Source: CAD feature listing. Evaluate the final solid. Frame: model axes, mm. A direction names the side the tool comes from. Round coordinates to 2 decimals unless told otherwise and drop trailing zeros. Order: outer loops, then holes, each group sorted by start corner. A loop starts at its lowest first (then second) coordinate and runs counter-clockwise, first axis right, second up. Notation, with made-up numbers: (-1.75, -20.75) -> (6.25, -20.75) arc R29 cw to (6.25, -0.75) -> close; hole circle Ø11 at (-14.75, 73.5). An arc over 180 degrees is marked (long way). Answer as CSV lines item,"result".
from build123d import *

# Parameters (mm, degrees)
CYLINDER007_R               = 5
CYLINDER007_DEPTH           = 5
COMPOUND003_PLACEMENT_ANGLE = 119
CYLINDER008_R               = 5
CYLINDER008_DEPTH           = 6
COMPOUND004_PLACEMENT_ANGLE = 119
CYLINDER006_R               = 5
CYLINDER006_DEPTH           = 6
CYLINDER004_R               = 2.5
CYLINDER004_DEPTH           = 12
COMPOUND_PLACEMENT_ANGLE    = 119
CYLINDER005_R               = 2.5
CYLINDER005_DEPTH           = 12
COMPOUND001_PLACEMENT_ANGLE = 241
CYLINDER003_R               = 2.5
CYLINDER003_DEPTH           = 12
BOX_W                       = 200
BOX_H                       = 100
BOX_DEPTH                   = 12
CYLINDER001_R               = 37.5
CYLINDER001_DEPTH           = 3
CYLINDER002_R               = 41
CYLINDER002_DEPTH           = 3
CYLINDER_R                  = 50
CYLINDER_DEPTH              = 12


with BuildPart() as compound003:
    # Cylinder007 → Cylinder007 (new body)
    with BuildSketch(Plane(origin=(0, -43.5, 0), x_dir=(1, 0, 0), z_dir=(0, 0, 1))):
        Circle(CYLINDER007_R)
    extrude(amount=CYLINDER007_DEPTH)


with BuildPart() as compound003_1:
    # Compound003 placement: moved
    add(compound003.part.rotate(Axis((0, 0, 0), (0, 0, 1)), COMPOUND003_PLACEMENT_ANGLE))


with BuildPart() as compound004:
    # Cylinder008 → Cylinder008 (new body)
    with BuildSketch(Plane(origin=(0, -43.5, 0), x_dir=(1, 0, 0), z_dir=(0, 0, 1))):
        Circle(CYLINDER008_R)
    extrude(amount=CYLINDER008_DEPTH)


with BuildPart() as compound004_1:
    # Compound004 placement: moved
    add(compound004.part.rotate(Axis((0, 0, 0), (0, 0, -1)), COMPOUND004_PLACEMENT_ANGLE))


with BuildPart() as compound005:
    # Cylinder006 → Cylinder006 (new body)
    with BuildSketch(Plane(origin=(0, -43.5, 0), x_dir=(1, 0, 0), z_dir=(0, 0, 1))):
        Circle(CYLINDER006_R)
    extrude(amount=CYLINDER006_DEPTH)

    # Compound005: union Compound003, Compound004
    add(compound003_1.part)
    add(compound004_1.part)


with BuildPart() as compound:
    # Cylinder004 → Cylinder004 (new body)
    with BuildSketch(Plane(origin=(0, -43.5, 0), x_dir=(1, 0, 0), z_dir=(0, 0, 1))):
        Circle(CYLINDER004_R)
    extrude(amount=CYLINDER004_DEPTH)


with BuildPart() as compound_1:
    # Compound placement: moved
    add(compound.part.rotate(Axis((0, 0, 0), (0, 0, 1)), COMPOUND_PLACEMENT_ANGLE))


with BuildPart() as compound001:
    # Cylinder005 → Cylinder005 (new body)
    with BuildSketch(Plane(origin=(0, -43.5, 0), x_dir=(1, 0, 0), z_dir=(0, 0, 1))):
        Circle(CYLINDER005_R)
    extrude(amount=CYLINDER005_DEPTH)


with BuildPart() as compound001_1:
    # Compound001 placement: moved
    add(compound001.part.rotate(Axis((0, 0, 0), (0, 0, 1)), COMPOUND001_PLACEMENT_ANGLE))


with BuildPart() as compound002:
    # Cylinder003 → Cylinder003 (new body)
    with BuildSketch(Plane(origin=(0, -43.5, 0), x_dir=(1, 0, 0), z_dir=(0, 0, 1))):
        Circle(CYLINDER003_R)
    extrude(amount=CYLINDER003_DEPTH)

    # Compound002: union Compound, Compound001
    add(compound_1.part)
    add(compound001_1.part)


with BuildPart() as cube:
    # Box → Box (new body)
    with BuildSketch(Plane(origin=(-100, 44, 0), x_dir=(1, 0, 0), z_dir=(0, 0, 1))):
        with Locations((100, 50)):
            Rectangle(BOX_W, BOX_H)
    extrude(amount=BOX_DEPTH)


with BuildPart() as cylinder001:
    # Cylinder001 → Cylinder001 (new body)
    with BuildSketch(Plane.XY):
        Circle(CYLINDER001_R)
    extrude(amount=CYLINDER001_DEPTH)


with BuildPart() as cut:
    # Cylinder002 → Cylinder002 (new body)
    with BuildSketch(Plane.XY):
        Circle(CYLINDER002_R)
    extrude(amount=CYLINDER002_DEPTH)

    # Cut: cut Cylinder001
    add(cylinder001.part, mode=Mode.SUBTRACT)


with BuildPart() as cut_1:
    # Cut placement: moved
    add(cut.part.moved(Location((0, 0, 9))))


with BuildPart() as xl30topbackflange100:
    # Cylinder → Cylinder (new body)
    with BuildSketch(Plane.XY):
        Circle(CYLINDER_R)
    extrude(amount=CYLINDER_DEPTH)

    # Cut001: cut Cut
    add(cut_1.part, mode=Mode.SUBTRACT)

    # Cut002: cut Cube
    add(cube.part, mode=Mode.SUBTRACT)

    # Cut003: cut Compound002
    add(compound002.part, mode=Mode.SUBTRACT)

    # Cut004: cut Compound005
    add(compound005.part, mode=Mode.SUBTRACT)


solid = xl30topbackflange100.part
1. Reachability of faces 1 (the cylindrical face through (-0.651, -38.543, 2.958)), 2 (the flat face through (18, -33.2, 9)), 3 (the cylindrical face through (35.55, 21.24, 8.45)) from +Z, -Z, +X, -X, +Y, -Y: full face, straight path, thin tool, end or side. Return the list, or none.
Results below:
face 1,"-Z"
face 2,"+Z"
face 3,"+Z, -Z"
2. Section query D-D on x = -20. Return loops of the section in (y, z).
Results below:
outline,"(-45.83, 0) -> (44, 0) -> (44, 12) -> (35.79, 12) -> (35.79, 9) -> (31.72, 9) -> (31.72, 12) -> (-31.72, 12) -> (-31.72, 9) -> (-35.79, 9) -> (-35.79, 12) -> (-45.83, 12) -> close"
3. Mould query, pull axis Y, two halves, no side actions, for faces 4 (the cylindrical face through (-35.675, 21.882, 8.958)), 5 (the cylindrical face through (-1.852, -49.966, 5.916)), 6 (the flat face through (-1, 1, 12)). Classes: released by +Y, released by -Y, zero draft, split by the parting line, or undercut.
Results below:
face 4,"undercut"
face 5,"split by the parting line"
face 6,"zero draft"
4. Section query C-C on z = 2. Return loops of the section in (x, y).
Results below:
outline,"(-23.75, 44) arc R50 ccw (long way) to (23.75, 44) -> close; hole circle Ø10 at (-38.05, 21.09); hole circle Ø10 at (0, -43.5); hole circle Ø10 at (38.05, 21.09)"
5. Pin query (flat end, axial travel): pin 1 (4 mm diameter, centred on x = -17, z = 4, fed in from -Y); pin 2 (2 mm diameter, centred on y = 22, z = 10, fed in from +X); pin 3 (5 mm diameter, centred on y = 13, z = 2.5, fed in from -X). Return the tip coordinate at first contact, or that it passes through.
Results below:
pin 1,"y = -47.7"
pin 2,"x = 45.38"
pin 3,"x = -48.89"
6. Line query: L1, parallel to Y at x = 19.5, z = 9.5; L2, parallel to Y at x = -10.5, z = 9.5; L3, parallel to Y at x = 0, z = 8.05. Output: solid intervals per line, ascending. Write a range as [from, to].
Results below:
L1,"[-46.04, -36.07], [-32.03, 32.03], [36.07, 44]"
L2,"[-48.89, -39.63], [-36, 36], [39.63, 44]"
L3,"[-50, -46], [-41, 44]"
7. Section query A-A on y = 0. Return loops of the section in (x, z), and give its area (3 significant figures).
Results below:
outline,"(-50, 0) -> (50, 0) -> (50, 12) -> (41, 12) -> (41, 9) -> (37.5, 9) -> (37.5, 12) -> (-37.5, 12) -> (-37.5, 9) -> (-41, 9) -> (-41, 12) -> (-50, 12) -> close"
area,"1,180 mm2"
8. Section query B-B on y = -43.5. Return loops of the section in (x, z).
Results below:
outline,"(-24.65, 0) -> (-5, 0) -> (-5, 6) -> (-2.5, 6) -> (-2.5, 12) -> (-24.65, 12) -> close; (2.5, 6) -> (5, 6) -> (5, 0) -> (24.65, 0) -> (24.65, 12) -> (2.5, 12) -> close"
